Autodesk Fusion 360 part; units mm, degrees
sketch "Sketch1" plane through (0, 0, 0) normal (0, 0, 1) x (1, 0, 0)
  line L0 (0, 0) -> (12.9082, -12.9082)
  line L1 (1.75, 0) -> (22.5, 0)
  line L2 (0, 0) -> (-12.9082, -12.9082)
  circle A0 centre (-12.2276, -12.2276) radius 0.9625
  circle A1 centre (12.2276, -12.2276) radius 0.9625
  circle A2 centre (0, 0) radius 6.675
  line L3 (-13.701, -10.7542) -> (-10.5388, -13.9165) construction
  line L4 (-12.9082, -11.5471) -> (-6.607, -0.9502)
  line L5 (-11.5471, -12.9082) -> (-0.9502, -6.607)
  line L6 (0, 1.75) -> (0, 22.5)
  line L7 (12.9082, -11.5471) -> (6.607, -0.9502)
  line L8 (11.5471, -12.9082) -> (0.9502, -6.607)
  dimension "d1" = 18.255
  dimension "d2" = 45
  dimension "d4" = -90
  dimension "d5" = 1.925
  dimension "d6" = 1.925
  dimension "d7" = 13.35
  dimension "d8" = 8
extrude "Extrude1" add sketch "Sketch1" along normal blind 2.58
sketch "Sketch2" plane through (0, 0, 2.58) normal (0, 0, 1) x (-1, 0, 0)
  line L0 (-12.9082, 11.5471) -> (-6.607, 0.9502)
  arc A0 (-6.607, 0.9502) -> (6.607, 0.9502) centre (0, 0) ccw
  line L1 (6.607, 0.9502) -> (12.9082, 11.5471)
  arc A1 (12.9082, 11.5471) -> (11.5471, 12.9082) centre (12.2276, 12.2276) ccw
  line L2 (11.5471, 12.9082) -> (0.9502, 6.607)
  arc A2 (0.9502, 6.607) -> (-0.9502, 6.607) centre (0, 0) ccw
  line L3 (-0.9502, 6.607) -> (-11.5471, 12.9082)
  arc A3 (-11.5471, 12.9082) -> (-12.9082, 11.5471) centre (-12.2276, 12.2276) ccw
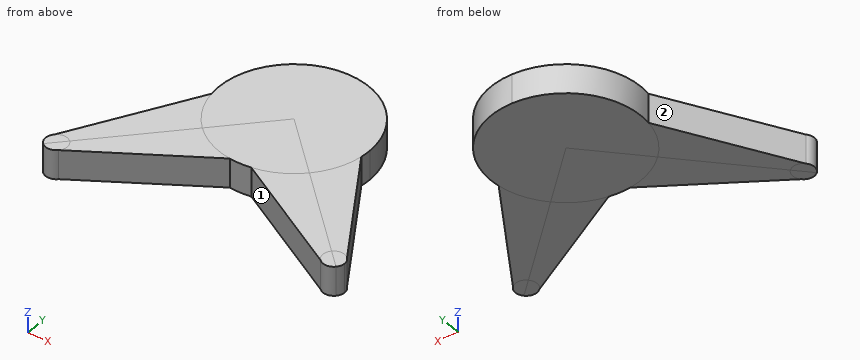
Could you check a few things on this model? Use its own coordinates, in mm. Face numbers are marked on the shaded views. Give positions to 0.01 mm unless a question says otherwise; leave off trailing zeros. Order: outer loops, then holes, each group sorted by start corner. A loop starts at its lowest first (then second) coordinate and runs counter-clockwise, first axis right, second up.
1. Suppose I cut it at A-A (y = -10.75). List the corners of the cut face in (x, z) for me, plus the area to 3 significant figures.
2. Suppose I cut it at D-D (y = 2.5). List the corners of the cut face in (x, z) for me.
3. We'd pull the mould along X, two halves only. Please class the marked faces 1 and 2: pulls with the +X half, pulls with the -X half, needs draft (parallel to the pull), parting line crosses it, or undercut.
4. Will this pin go through, and if not, where does the flat tip stop? P1, Ø1.5, axis at y = -4.5, z = 1, coming from the +X side.
5. Suppose I cut it at C-C (x = -8.25). List the corners of the cut face in (y, z) for me.
6. I need wall thicknesses on L1, parallel to X at y = -8.5, z = 1.75; L2, parallel to X at y = -11, z = 1.7; L3, parallel to X at y = 2.5, z = 0.2. Which ranges of each line are inside material? Lowest first, please.
Solved:
1. outline: (-12.43, 0) - (-7.92, 0) - (-7.92, 2.58) - (-12.43, 2.58) - close; (7.92, 0) - (12.43, 0) - (12.43, 2.58) - (7.92, 2.58) - close
1. area: 23.3 mm2
2. outline: (-6.19, 0) - (6.19, 0) - (6.19, 2.58) - (-6.19, 2.58) - close
3. face 1: undercut
3. face 2: pulls with the -X half
4. P1: stops at x = 9.16
5. outline: (-10.95, 0) - (-3.71, 0) - (-3.71, 2.58) - (-10.95, 2.58) - close
6. L1: x = -11.1 to -4.13, 4.13 to 11.1
6. L2: x = -12.58 to -8.34, 8.34 to 12.58
6. L3: x = -6.19 to 6.19
